```python
from build123d import *

# Parameters (mm, degrees)
SKETCH1_W                = 25.5
SKETCH1_H                = 25.5
SKETCH1_W_2              = 23.1
SKETCH1_H_2              = 23.1
BOSS_EXTRUDE1_DEPTH      = 149
F_6_0_6_DIAMETER_HOLE5_D = 6
F_6_0_6_DIAMETER_HOLE7_D = 6


with BuildPart() as part:
    # Sketch1 → Boss-Extrude1 (new body)
    with BuildSketch(Plane.XY):
        Rectangle(SKETCH1_W, SKETCH1_H)
        Rectangle(SKETCH1_W_2, SKETCH1_H_2, mode=Mode.SUBTRACT)
    extrude(amount=BOSS_EXTRUDE1_DEPTH)

    # Ø6.0 (6) Diameter Hole5 (through all)
    with Locations(Plane(origin=(-0.05, -21.75, 65), x_dir=(0, 0, -1), z_dir=(0, -1, 0))):
        with Locations((0, 0)):
            Hole(F_6_0_6_DIAMETER_HOLE5_D / 2)

    # Ø6.0 (6) Diameter Hole7 (through all)
    with Locations(Plane.ZY.offset(12.75)):
        with Locations((37.2, 0.15), (87.2, 0.15), (137.2, 0.15)):
            Hole(F_6_0_6_DIAMETER_HOLE7_D / 2)


solid = part.part
```
Check sheet for the modelled part. Datum: model origin and axes. Units: mm. A direction names the side the tool comes from. Give positions to 0.01 mm unless a question says otherwise; leave off trailing zeros. Order: outer loops, then holes, each group sorted by start corner. A loop starts at its lowest first (then second) coordinate and runs counter-clockwise, first axis right, second up. Notation, with made-up numbers: (51.25, 20) -> (70.25, 20) arc R19 ccw to (70.25, 27) -> close; hole circle Ø3 at (54, -0.75). An arc over 180 degrees is marked (long way). Return JSON: item names as keys, results as strings.
1. Set-up check for faces 5 (the cylindrical face through (12.16, 1.05, 34.34)), 6 (the flat face through (11.55, 0, 73)): record each of +Z, -Z, +X, -X, +Y, -Y from which the full face is reachable in a straight line by a thin tool's end or side.
From the geometry:
{"face 5": "+X, -X", "face 6": "+Z, -Z"}
2. Material ranges on probe 1 along Y at (x, z) = (-1.75, 10); probe 2 along Y at (x, z) = (12.5, 87.2), recorded low to high. Write a range as [from, to].
From the geometry:
{"probe 1": "[-12.75, -11.55], [11.55, 12.75]", "probe 2": "[-12.75, -2.85], [3.15, 12.75]"}
3. Cross-section at B-B, the plane y = 0.15. Count the separate pieces of the cut face and the enclosed holes in it, plus the area to 3 significant figures.
From the geometry:
{"separate pieces": "8", "enclosed holes": "0", "area": "314 mm^2"}
4. Mould release check, pull along Y, two halves, no side actions. Record for faces 1 (the cylindrical face through (-12.14, 1.05, 84.34)), 2 (the flat face through (-1, -12, 149)), 3 (the flat face through (0, -12.75, 73)), 4 (the flat face through (-11.55, 0, 73)): +Y half, -Y half, draft (parallel to the pull), parting line (faces both ways), or undercut.
From the geometry:
{"face 1": "undercut", "face 2": "draft", "face 3": "-Y half", "face 4": "undercut"}
5. Cross-section at A-A, the plane x = -6.25. Record the cut outline in (y, z), plus the area to 3 significant figures.
From the geometry:
{"outline": "(-12.75, 0) -> (-11.55, 0) -> (-11.55, 149) -> (-12.75, 149) -> close; (11.55, 0) -> (12.75, 0) -> (12.75, 149) -> (11.55, 149) -> close", "area": "358 mm^2"}
6. Cross-section at D-D, the plane x = -0.05. Record the cut outline in (y, z), plus the area to 3 significant figures.
From the geometry:
{"outline": "(-12.75, 0) -> (-11.55, 0) -> (-11.55, 62) -> (-12.75, 62) -> close; (-12.75, 68) -> (-11.55, 68) -> (-11.55, 149) -> (-12.75, 149) -> close; (11.55, 0) -> (12.75, 0) -> (12.75, 62) -> (11.55, 62) -> close; (11.55, 68) -> (12.75, 68) -> (12.75, 149) -> (11.55, 149) -> close", "area": "343 mm^2"}
7. Go/stop test with a flat-tipped pin: P1, Ø5, axis at y = 0.15, z = 37.2, coming from the -X side. Record where the tip stops, or that it passes through.
From the geometry:
{"P1": "through"}
8. Cross-section at C-C, the plane z = 87.2. Record the cut outline in (x, y), plus the area to 3 significant figures.
From the geometry:
{"outline": "(-12.75, -12.75) -> (12.75, -12.75) -> (12.75, -2.85) -> (11.55, -2.85) -> (11.55, -11.55) -> (-11.55, -11.55) -> (-11.55, -2.85) -> (-12.75, -2.85) -> close; (-12.75, 3.15) -> (-11.55, 3.15) -> (-11.55, 11.55) -> (11.55, 11.55) -> (11.55, 3.15) -> (12.75, 3.15) -> (12.75, 12.75) -> (-12.75, 12.75) -> close", "area": "102 mm^2"}
